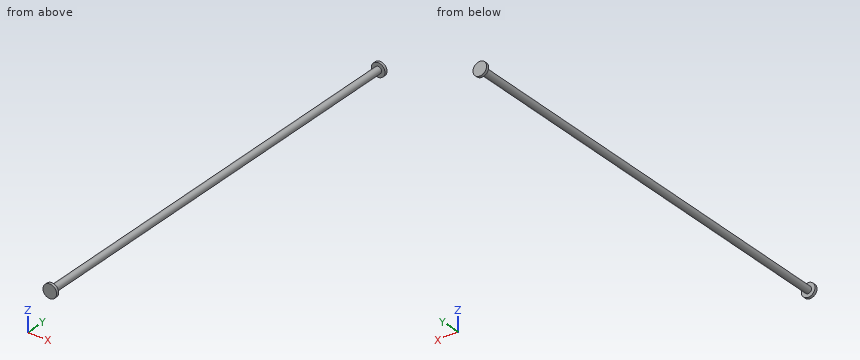
from build123d import *

# Parameters (mm, degrees)
SKETCH1_R           = 2.5
BOSS_EXTRUDE1_DEPTH = 320
SKETCH2_R           = 5
BOSS_EXTRUDE2_DEPTH = 2
SKETCH3_R           = 5
BOSS_EXTRUDE3_DEPTH = 2


with BuildPart() as part:
    # Sketch1 → Boss-Extrude1 (new body)
    with BuildSketch(Plane(origin=(0, 0, 0), x_dir=(1, 0, 0), z_dir=(0, 1, 0))):
        Circle(SKETCH1_R)
    extrude(amount=BOSS_EXTRUDE1_DEPTH)

    # Sketch2 → Boss-Extrude2 (add)
    with BuildSketch(Plane.XZ):
        Circle(SKETCH2_R)
    extrude(amount=BOSS_EXTRUDE2_DEPTH)

    # Sketch3 → Boss-Extrude3 (add)
    with BuildSketch(Plane(origin=(0, 320, 0), x_dir=(1, 0, 0), z_dir=(0, 1, 0))):
        Circle(SKETCH3_R)
    extrude(amount=BOSS_EXTRUDE3_DEPTH)


solid = part.part
Part model, mm, in its own coordinate system. Round coordinates to 2 decimals unless told otherwise and drop trailing zeros. Order: outer loops, then holes, each group sorted by start corner. A loop starts at its lowest first (then second) coordinate and runs counter-clockwise, first axis right, second up. Notation, with made-up numbers: (-22.75, -14.5) -> (2.25, -14.5) arc R19 ccw to (2.25, 16.5) -> close; hole circle Ø6 at (22.25, -38). An arc over 180 degrees is marked (long way). Put each result on its own line as item: value.
Q1. Band-saw the part on B-B (x = 0). Give the cut face in (y, z), and give its area (3 significant figures).
From the geometry:
outline: (-2, -5) -> (0, -5) -> (0, -2.5) -> (320, -2.5) -> (320, -5) -> (322, -5) -> (322, 5) -> (320, 5) -> (320, 2.5) -> (0, 2.5) -> (0, 5) -> (-2, 5) -> close
area: 1,640 mm2
Q2. Band-saw the part on A-A (z = 0). Give the cut face in (x, y), and give its area (3 significant figures).
From the geometry:
outline: (-5, -2) -> (5, -2) -> (5, 0) -> (2.5, 0) -> (2.5, 320) -> (5, 320) -> (5, 322) -> (-5, 322) -> (-5, 320) -> (-2.5, 320) -> (-2.5, 0) -> (-5, 0) -> close
area: 1,640 mm2
Q3. Band-saw the part on C-C (y = 245). Give the cut face in (x, z).
From the geometry:
outline: circle Ø5 at (0, 0)
Q4. Pin check, flat tips, straight feed: pin 1 Ø1 at (y, z) = (118.5, -1.5) entering from +X; pin 2 Ø6 at (x, y) = (-2, 264.5) entering from +Z; pin 3 Ø6 at (x, y) = (-3, 240) entering from -Z. Stop position of each tip, or through.
From the geometry:
pin 1: stops at x = 2.29
pin 2: stops at z = 2.5
pin 3: stops at z = -2.5
Q5. Wall check: line 1 (Y direction, x = 3.75, z = -2.75); line 2 (X direction, y = 236, z = -0.5); line 3 (Z direction, x = 2, y = 56.5). Give the ranges that are in metal, low to high. Write a range as [from, to].
From the geometry:
line 1: y = [-2, 0], [320, 322]
line 2: x = [-2.45, 2.45]
line 3: z = [-1.5, 1.5]
